from build123d import *

# Parameters (mm, degrees)
CONG_1_R = 1.5
CONG_2_R = 10


with BuildPart() as part:
    # Esquisse1 → Révolution1 (revolve)
    with BuildSketch(Plane.XY, mode=Mode.PRIVATE) as r_volution1_sk:
        Polygon((59.159659942, -7), (62.9, -7), (62.9, 0), (54, 0), (54, 5), (0, 5), (0, 0), (0, -6.5), (47, -6.5), (47, -31), (56, -31), (56.987393732, -23.5), (54.514003722, -23.5), (54.514003722, -19.5), (57.514003722, -19.5), (58.106439961, -15), (55.633049952, -15), (55.633049952, -11), (58.633049952, -11), align=None)
    revolve(r_volution1_sk.sketch.rotate(Axis((0, 0, 0), (0, 1, 0)), 90), axis=Axis((0, 0, 0), (0, 1, 0)))

    # Congé1
    cong_1_edges = [part.edges().sort_by_distance(p)[0] for p in [
        (0, -11, 55.633049952),
        (0, -15, 55.633049952),
        (0, -19.5, 54.514003722),
        (0, -23.5, 54.514003722),
    ]]
    fillet(cong_1_edges, radius=CONG_1_R)

    # Congé2
    cong_2_edges = [part.edges().sort_by_distance(p)[0] for p in [
        (0, -6.5, 47),
    ]]
    fillet(cong_2_edges, radius=CONG_2_R)


solid = part.part
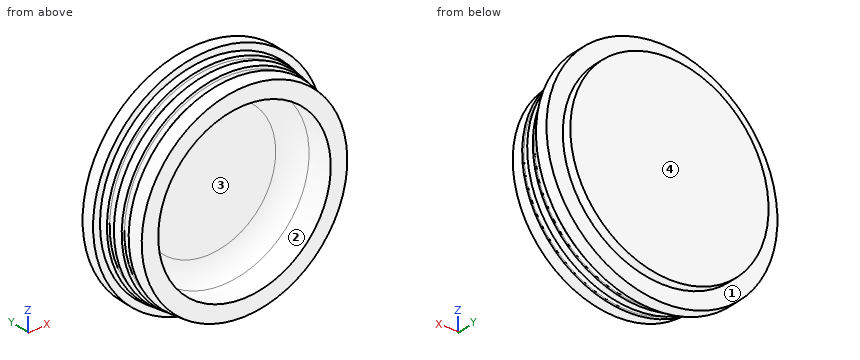
Here's how the part is built. I have some questions about the finished solid (model axes, mm). Face numbers are marked on the shaded views. A direction names the side the tool comes from. Coordinates: 2 decimals unless noted, no trailing zeros. Loops run counter-clockwise (first coordinate to the right, second up) from the corner with the lowest first, then second, coordinate; pieces in that order, holes last. Notation, with made-up numbers: (11.25, -37) -> (66.25, -37) arc R18 ccw to (66.25, -14) -> close; hole circle Ø6 at (16, -20). An arc over 180 degrees is marked (long way). Use one line per item in the form item = value. Start each with the question number.
(1) Please list where these lines run through material, in increasing order: line 1 along Y through (x, z) = (-16, 8); line 2 along X through (y, z) = (-29, 8); line 3 along X through (y, z) = (-22.5, 0).
(2) If we section it at A-A (y = -27.5): Please give me the cut outline in (x, z).
(3) Will these pins go through, and if not, where does the flat tip stop? pin 1 (6 mm diameter, centred on x = 11, y = -8, fed in from +Z); pin 2 (1 mm diameter, centred on x = 17.5, y = -3.5, fed in from -Z); pin 3 (8 mm diameter, centred on y = -5.5, z = -38, fed in from -X).
(4) On a 3-axis mill with a long thin cutter (end or side, diameter ignored), from which of +Z, -Z, +X, -X, +Y, -Y can I reach the whole of each face in a straight line? I mean the marked faces 3 and 4. Say none if no direction works.
(5) We'd pull the mould along Z, two halves only. Please class the marked faces 1 and 2: pulls with the +Z half, pulls with the -Z half, needs draft (parallel to the pull), parting line crosses it, or undercut.
(6) If we section it at B-B (y = -18): Please give me the cut outline in (x, z), then the cut area to 3 significant figures.
Verdict:
q1.line_1 = -6.5 to 5
q1.line_2 = -55.69 to -46.31, 46.31 to 55.69
q1.line_3 = -54.6 to -47, 47 to 54.6
q2.outline = circle Ø112.92 at (0, 0); hole circle Ø94 at (0, 0)
q3.pin_1 = 62.37
q3.pin_2 = -60.56
q3.pin_3 = -52.92
q4.face_3 = -Y
q4.face_4 = +Z, -Z, +X, -X, +Y
q5.face_1 = needs draft
q5.face_2 = undercut
q6.outline = circle Ø115.42 at (0, 0); hole circle Ø94 at (0, 0)
q6.area = 3,520 mm²
